CAD build for the part. Positions are in the model's coordinates, mm. A direction names the side the tool comes from. Coordinates: 2 decimals unless noted, no trailing zeros. Write each loop counter-clockwise with the first axis right and the second up, starting at its lowest first coordinate (ties: lowest second). Pieces come first, ordered by that corner, then holes. Notation, with made-up numbers: (-27, -19.5) - (15, -19.5) arc R21 cw to (15, 12.5) - close; hole circle Ø11 at (14, 70). An arc over 180 degrees is marked (long way). One line per question, with ' | ' between items. Start each with the question number.
1. Two-plate mould, pull along X, no slides. Class faces 1 (the flat face through (37, 1, 9)), 2 (the flat face through (74, 5, 4)), 3 (the flat face through (37, 7, 2)): +X half, -X half, draft (parallel to the pull), parting line (faces both ways), or undercut.
2. Band-saw the part on B-B, the plane y = 3. Write the cut outline in (x, z).
3. Flat gauge pins, fed straight in: P1, Ø3.5, axis at x = 67.5, y = 6.5, coming from the +Z side; P2, Ø2, axis at x = 53, z = 4, coming from the +Y side. Where does each tip first touch, or does it go through?
4. Which spindle directions (+Z, -Z, +X, -X, +Y, -Y) get a long thin tool onto all of the face, cutting with end or side? Do faces 4 (the flat face through (36, 6, 0)), 5 (the cylindrical face through (9.717, 9.647, 4.535)). Say none if no direction does.
5. Probe line 1 (X direction, y = 5.25, z = 6.5); line 2 (Y direction, x = 67.5, z = 5.5); line 3 (X direction, y = 8, z = 7.25). List the from-to ranges inside material, lowest first.
6. Band-saw the part on D-D, the plane y = 9.75. Write the cut outline in (x, z), then the cut area to 3 significant figures.
7. Band-saw the part on A-A, the plane z = 5.5. Write the cut outline in (x, y), then the cut area to 3 significant figures.
8. Band-saw the part on C-C, the plane x = 46. Write the cut outline in (y, z), then the cut area to 3 significant figures.
from build123d import *

# Parameters (mm, degrees)
SKETCH_1_W        = 9
SKETCH_1_H        = 9
SKETCH_1_R        = 1.1
EXTRUDE_1_DEPTH   = 7
EXTRUDE_1_2_DEPTH = 7
SKETCH_1_3_W      = 52
SKETCH_1_3_H      = 9
EXTRUDE_2_DEPTH   = 2
EXTRUDE_3_DEPTH   = 9
FILLET_1_R        = 4.5


with BuildPart() as part:
    # Sketch 1 → Extrude 1 (new body)
    with BuildSketch(Plane.XY):
        with Locations((6.5, 6.5)):
            Rectangle(SKETCH_1_W, SKETCH_1_H)
        with Locations((6.5, 6.5)):
            Circle(SKETCH_1_R, mode=Mode.SUBTRACT)
    extrude(amount=EXTRUDE_1_DEPTH)



with BuildPart() as body_2:
    # Sketch 1 → Extrude 1 2 (new body)
    with BuildSketch(Plane.XY):
        with Locations((67.5, 6.5)):
            Rectangle(SKETCH_1_W, SKETCH_1_H)
        with Locations((67.5, 6.5)):
            Circle(SKETCH_1_R, mode=Mode.SUBTRACT)
    extrude(amount=EXTRUDE_1_2_DEPTH)


with BuildPart() as part_1:
    add(part.part)

    add(body_2.part)  # Extrude 2 merges body 2
    # Sketch 1_3 → Extrude 2 (add)
    with BuildSketch(Plane.XY):
        with Locations((37, 6.5)):
            Rectangle(SKETCH_1_3_W, SKETCH_1_3_H)
    extrude(amount=EXTRUDE_2_DEPTH)

    # Sketch 1_4 → Extrude 3 (add)
    with BuildSketch(Plane.XY):
        Polygon((0, 11), (0, 0), (74, 0), (74, 11), (72, 11), (72, 2), (63, 2), (11, 2), (2, 2), (2, 11), align=None)
    extrude(amount=EXTRUDE_3_DEPTH)

    # Fillet 1
    fillet_1_edges = [part_1.edges().sort_by_distance(p)[0] for p in [
        (11, 11, 4.5),
        (63, 11, 4.5),
    ]]
    fillet(fillet_1_edges, radius=FILLET_1_R)


solid = part_1.part
Filled in:
1) face 1: draft | face 2: +X half | face 3: undercut
2) outline: (0, 0) - (74, 0) - (74, 9) - (72, 9) - (72, 7) - (63, 7) - (63, 2) - (11, 2) - (11, 7) - (2, 7) - (2, 9) - (0, 9) - close
3) P1: stops at z = 7 | P2: stops at y = 2
4) face 4: -Z, +X, -X, +Y, -Y | face 5: +Z, +Y
5) line 1: x = 0 to 11, 63 to 74 | line 2: y = 0 to 5.4, 7.6 to 11 | line 3: x = 0 to 2, 72 to 74
6) outline: (0, 0) - (74, 0) - (74, 9) - (72, 9) - (72, 7) - (64.39, 7) - (64.39, 2) - (9.61, 2) - (9.61, 7) - (2, 7) - (2, 9) - (0, 9) - close | area: 252 mm²
7) outline: (0, 0) - (74, 0) - (74, 11) - (67.5, 11) arc R4.5 ccw to (63, 6.5) - (63, 2) - (11, 2) - (11, 6.5) arc R4.5 ccw to (6.5, 11) - (0, 11) - close; hole circle Ø2.2 at (6.5, 6.5); hole circle Ø2.2 at (67.5, 6.5) | area: 330 mm²
8) outline: (0, 0) - (11, 0) - (11, 2) - (2, 2) - (2, 9) - (0, 9) - close | area: 36.0 mm²
